Source: three-view drawing plus pictorial views. Frame: mm from the lowest corner of the part. Round coordinates to 2 decimals unless told otherwise and drop trailing zeros. Order: outer loops, then holes, each group sorted by start corner. A loop starts at its lowest first (then second) coordinate and runs counter-clockwise, first axis right, second up. Notation, with made-up numbers: (3, 75) -> (21, 75) arc R22 ccw to (21, 84) -> close; hole circle Ø1 at (17.5, -36.5). An arc over 180 degrees is marked (long way). Use a Markdown table: item, result.
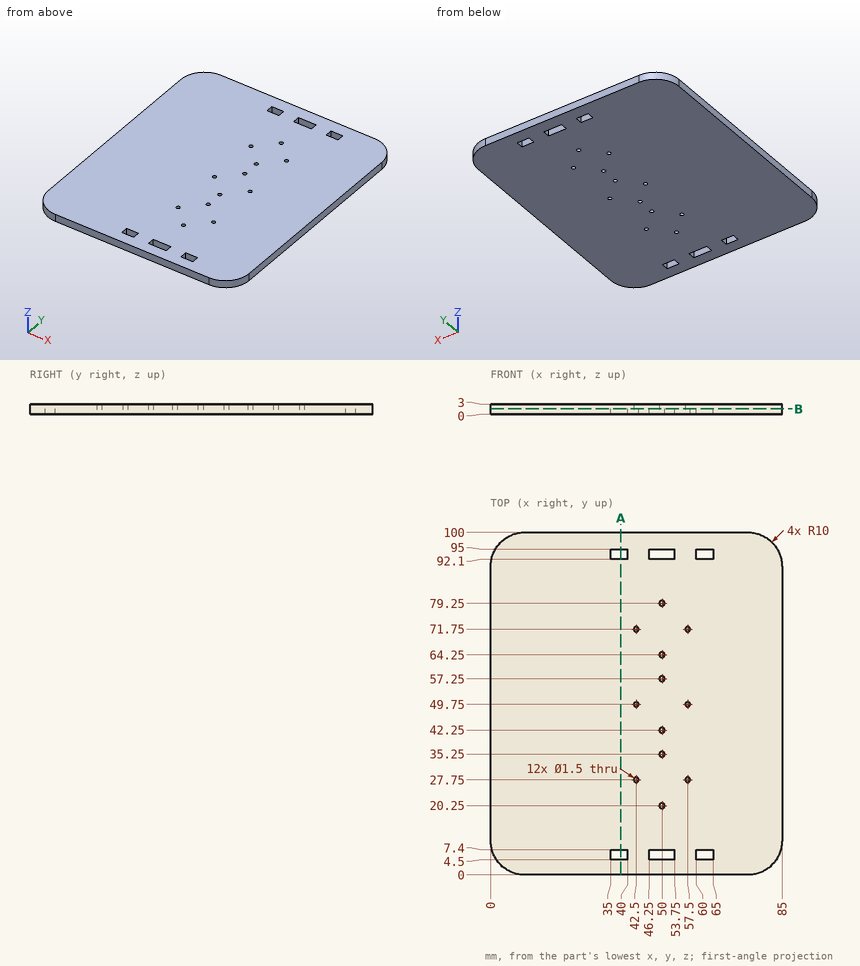
1) Cut plane B-B on z = 1.6. Count the separate pieces of the cut face and the enclosed holes in it, and give its area (3 significant figures).
Results found:
| item | result |
|---|---|
| separate pieces | 1 |
| enclosed holes | 18 |
| area | 8,290 mm² |
2) Pin query (flat end, axial travel): pin 1 Ø0.9 at (y, z) = (93, 1) entering from -X; pin 2 Ø1.5 at (y, z) = (5.5, 1.5) entering from +X; pin 3 Ø0.9 at (y, z) = (93, 2) entering from +X. Return the tip coordinate at first contact, or that it passes through.
Results found:
| item | result |
|---|---|
| pin 1 | stops at x = 0.33 |
| pin 2 | stops at x = 84.27 |
| pin 3 | stops at x = 84.67 |
3) Line query: L1, parallel to Y at x = 42.5, z = 1.65; L2, parallel to X at y = 57.25, z = 0.75; L3, parallel to X at y = 27.75, z = 2.05. Output: solid intervals per line, ascending. Write a range as [from, to].
Results found:
| item | result |
|---|---|
| L1 | y = [0, 27], [28.5, 49], [50.5, 71], [72.5, 100] |
| L2 | x = [0, 49.25], [50.75, 85] |
| L3 | x = [0, 41.75], [43.25, 56.75], [58.25, 85] |
4) Cut plane A-A on x = 38. Return loops of the section in (y, z).
Results found:
| item | result |
|---|---|
| outline | (0, 0) -> (4.5, 0) -> (4.5, 3) -> (0, 3) -> close; (7.4, 0) -> (92.1, 0) -> (92.1, 3) -> (7.4, 3) -> close; (95, 0) -> (100, 0) -> (100, 3) -> (95, 3) -> close |
